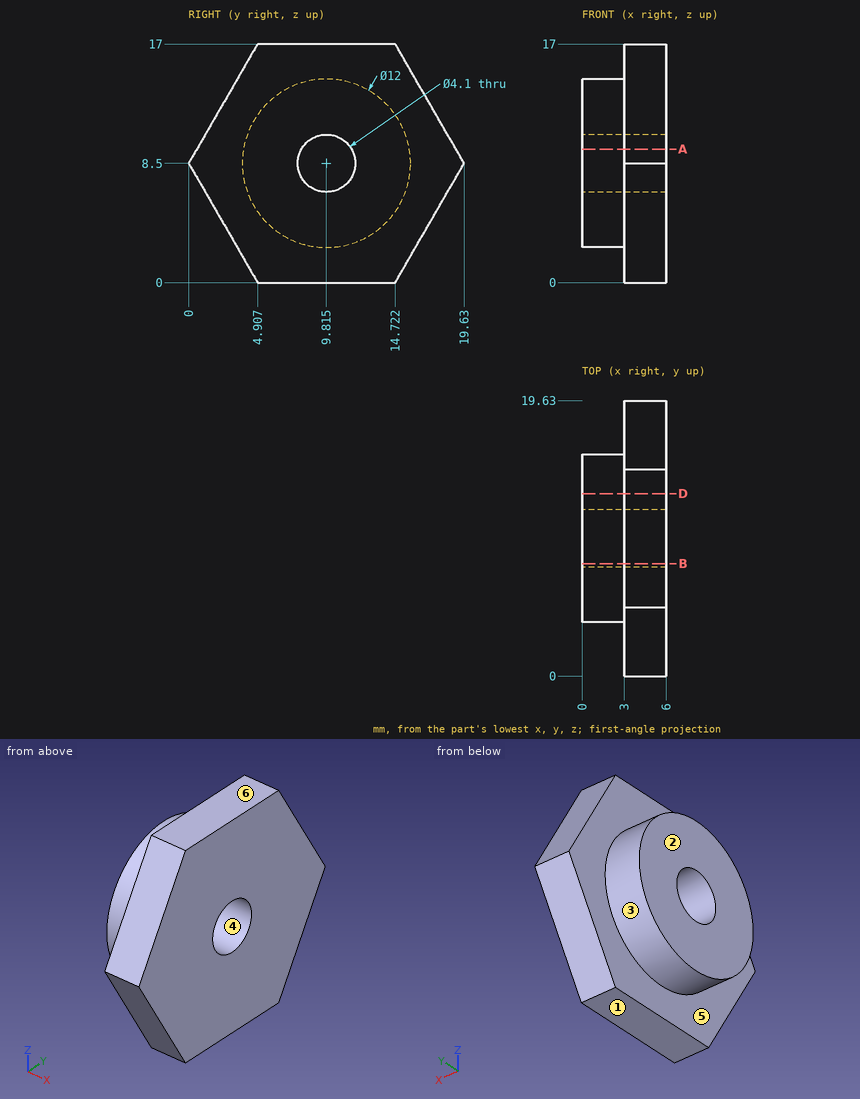
Input: dimensioned drawing with shaded views. Units: mm. Origin: part minimum x, y, z. A direction names the side the tool comes from. Coordinates: 2 decimals unless noted, no trailing zeros. Order: outer loops, then holes, each group sorted by start corner. A loop starts at its lowest first (then second) coordinate and runs counter-clockwise, first axis right, second up. Notation, with made-up numbers: (45, 24) - (63, 24) arc R20 ccw to (63, 38) - close; hole circle Ø11 at (73, -20). An arc over 180 degrees is marked (long way). Return JSON: item names as keys, results as strings. Group by question number.
1. Cut plane A-A (z = 9.5). Output: boundary loops of the cut face in (x, y) (1 decimal).
2. Cut plane D-D (y = 13). Output: boundary loops of the cut face in (x, z) (1 decimal).
3. Pull-direction query (Z, two-part tool) for the marked faces 1, 2, 3 and 4; classes: pulls with the +Z half, pulls with the -Z half, needs draft (parallel to the pull), parting line crosses it, or undercut.
4. Cut plane B-B (y = 8). Output: boundary loops of the cut face in (x, z).
5. Set-up query: the marked faces 5 and 6. Return all of +Z, -Z, +X, -X, +Y, -Y with unobstructed straight access to the full face (end or side cutting, diameter ignored); none if empty.
6. Pin query (flat end, axial travel): pin 1 (3 mm diameter, centred on x = 3.5, z = 2.5, fed in from +Y). Return the tip coordinate at first contact, or that it passes through.
7. Material intervals for line 1 along X through (y, z) = (7.75, 14.25); line 2 along Z through (x, y) = (5.7, 9.5) (1 decimal); line 3 along Z through (x, y) = (1.35, 11.5) (1 decimal), sorted ascending. Write a range as [from, to].
Resolved:
{
 "1": {"outline": "(0, 3.9) - (3, 3.9) - (3, 0.6) - (6, 0.6) - (6, 8) - (0, 8) - close; (0, 11.6) - (6, 11.6) - (6, 19.1) - (3, 19.1) - (3, 15.7) - (0, 15.7) - close"},
 "2": {"outline": "(0, 3.4) - (3, 3.4) - (3, 0) - (6, 0) - (6, 17) - (3, 17) - (3, 13.6) - (0, 13.6) - close"},
 "3": {"face 1": "pulls with the -Z half", "face 2": "needs draft", "face 3": "parting line crosses it", "face 4": "undercut"},
 "4": {"outline": "(0, 2.78) - (3, 2.78) - (3, 0) - (6, 0) - (6, 7.55) - (0, 7.55) - close; (0, 9.45) - (6, 9.45) - (6, 17) - (3, 17) - (3, 14.22) - (0, 14.22) - close"},
 "5": {"face 5": "-X", "face 6": "+Z, +X, -X, +Y, -Y"},
 "6": {"pin 1": "stops at y = 17.03"},
 "7": {"line 1": "x = [3, 6]", "line 2": "z = [0, 6.5], [10.5, 17]", "line 3": "z = [2.7, 7.3], [9.7, 14.3]"}
}
